Here's how the part is built. I have some questions about the finished solid (model axes, mm). Give positions to 0.01 mm unless a question says otherwise; leave off trailing zeros. Write each loop counter-clockwise with the first axis right and the second up, starting at its lowest first coordinate (ties: lowest second). Pieces come first, ordered by that corner, then holes. Notation, with made-up numbers: (84.25, 5.5) -> (97.25, 5.5) arc R21 ccw to (97.25, 21.5) -> close; hole circle Ø5 at (-7.5, -39.5). An arc over 180 degrees is marked (long way). Answer as CSV lines item,"result". Start each with the question number.
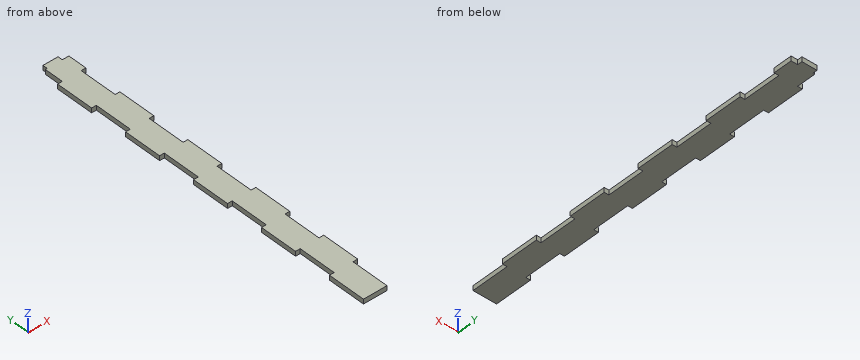
Autodesk Fusion 360 part; units mm, degrees
sketch "スケッチ1" plane through (0, 0, 0) normal (0, 0, 1) x (1, 0, 0)
  line L0 (20.0472, -16.9044) -> (20.0472, -26.9043)
  line L1 (20.0472, -26.9043) -> (17.5473, -26.9043)
  line L2 (17.5473, -26.9043) -> (17.5473, -46.9043)
  line L3 (17.5473, -46.9043) -> (20.0472, -46.9043)
  line L4 (20.0472, -46.9043) -> (20.0472, -66.9043)
  line L5 (20.0472, -66.9043) -> (17.5473, -66.9043)
  line L6 (17.5473, -66.9043) -> (17.5473, -86.9043)
  line L7 (17.5473, -86.9043) -> (20.0472, -86.9043)
  line L8 (20.0472, -86.9043) -> (20.0472, -106.9043)
  line L9 (20.0472, -106.9043) -> (17.5473, -106.9043)
  line L10 (17.5473, -106.9043) -> (17.5473, -126.9043)
  line L11 (17.5473, -126.9043) -> (20.0472, -126.9043)
  line L12 (20.0472, -126.9043) -> (20.0472, -146.9043)
  line L13 (20.0472, -146.9043) -> (17.5473, -146.9043)
  line L14 (17.5473, -146.9043) -> (17.5473, -166.9043)
  line L15 (17.5473, -166.9043) -> (20.0472, -166.9043)
  line L16 (20.0472, -166.9043) -> (20.0472, -186.9045)
  line L17 (20.0472, -186.9045) -> (17.5473, -186.9045)
  line L18 (17.5473, -186.9045) -> (17.5473, -206.9043)
  spline S0 degree 3 poles (17.5473, -206.9043) (17.5473, -206.9046) (30.0472, -206.9046) (30.0473, -206.9046) knots 19 19 19 19 20 20 20 20
  line L19 (30.0473, -206.9046) -> (30.0473, -186.9045)
  line L20 (30.0473, -186.9045) -> (32.5472, -186.9045)
  line L21 (32.5472, -186.9045) -> (32.5472, -166.9043)
  line L22 (32.5472, -166.9043) -> (30.0473, -166.9043)
  line L23 (30.0473, -166.9043) -> (30.0473, -146.9043)
  line L24 (30.0473, -146.9043) -> (32.5472, -146.9043)
  line L25 (32.5472, -146.9043) -> (32.5472, -126.9043)
  line L26 (32.5472, -126.9043) -> (30.0473, -126.9043)
  line L27 (30.0473, -126.9043) -> (30.0473, -106.9043)
  line L28 (30.0473, -106.9043) -> (32.5472, -106.9043)
  line L29 (32.5472, -106.9043) -> (32.5472, -86.9043)
  line L30 (32.5472, -86.9043) -> (30.0473, -86.9043)
  line L31 (30.0473, -86.9043) -> (30.0473, -66.9043)
  line L32 (30.0473, -66.9043) -> (32.5472, -66.9043)
  line L33 (32.5472, -66.9043) -> (32.5472, -46.9043)
  line L34 (32.5472, -46.9043) -> (30.0473, -46.9043)
  line L35 (30.0473, -46.9043) -> (30.0473, -26.9043)
  line L36 (30.0473, -26.9043) -> (32.5472, -26.9043)
  line L37 (32.5472, -26.9043) -> (32.5472, -16.9044)
  line L38 (32.5472, -16.9044) -> (29.0473, -16.9044)
  line L39 (29.0473, -16.9044) -> (29.0473, -14.4045)
  line L40 (29.0473, -14.4045) -> (21.0473, -14.4045)
  line L41 (21.0473, -14.4045) -> (21.0473, -16.9044)
  line L42 (21.0473, -16.9044) -> (20.0472, -16.9044)
extrude "押し出し1" add sketch "スケッチ1" along normal blind 2.5
Item 1: If I drill on line 1 (Y direction, x = 31.5, z = 1.7); line 2 (Y direction, x = 20, z = 1.85); line 3 (X direction, y = -95, z = 2.05), over which ranges is the centre line in solid material (lowest first)? Write a range as [from, to].
Item 2: If we section it at A-A (y = -53): Please give me the cut outline in (x, z), and give its area (4 significant figures).
Item 3: I'm going to push flat-ended pins straight in: pin 1 (0.8 mm diameter, centred on x = 31.5, z = 1.5, fed in from +Y); pin 2 (0.8 mm diameter, centred on y = -79.5, z = 1, fed in from +X). Where does each tip first touch, or does it pass through?
Final values:
1,line 1,"[-186.9, -166.9], [-146.9, -126.9], [-106.9, -86.9], [-66.9, -46.9], [-26.9, -16.9]"
1,line 2,"[-206.9, -186.9], [-166.9, -146.9], [-126.9, -106.9], [-86.9, -66.9], [-46.9, -26.9]"
1,line 3,"[20.05, 32.55]"
2,outline,"(20.05, 0) -> (32.55, 0) -> (32.55, 2.5) -> (20.05, 2.5) -> close"
2,area,"31.25 mm2"
3,pin 1,"y = -16.9"
3,pin 2,"x = 30.05"
